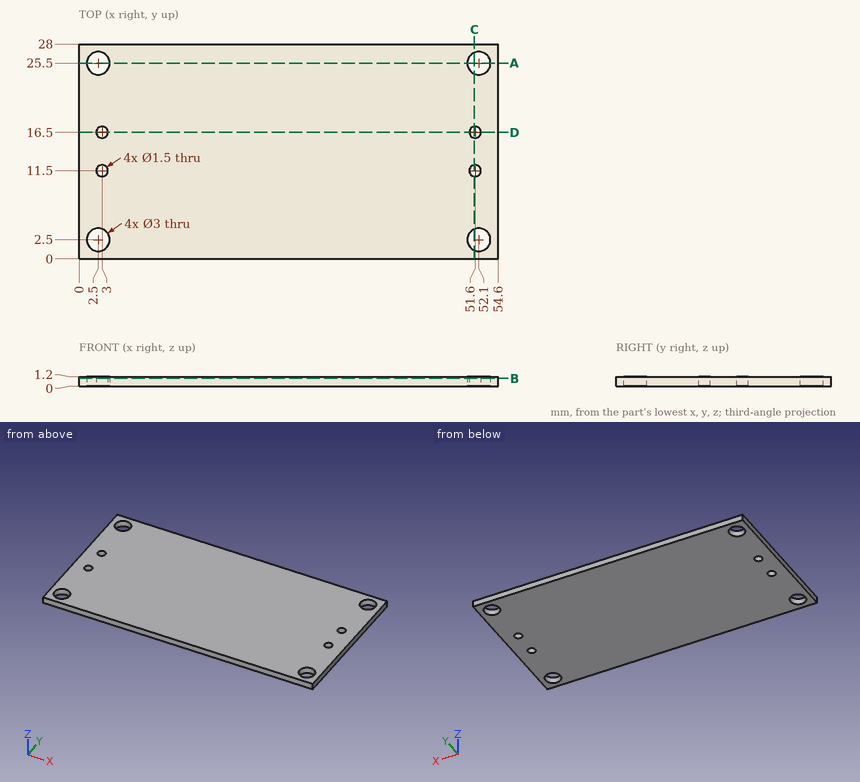
The figure shows three views and two pictorial views of one solid part (mm, origin at its lowest corner). Answer the questions. Give positions to 0.01 mm unless a question says otherwise; leave off trailing zeros. Write each loop counter-clockwise with the first axis right and the second up, starting at its lowest first coordinate (ties: lowest second). Pieces come first, ordered by that corner, then holes. Notation, with made-up numbers: (-30, 48) - (20, 48) arc R20 ccw to (20, 76) - close; hole circle Ø7 at (56.5, 14.25). An arc over 180 degrees is marked (long way). Use one line per item in the form item = value. Start each with the question number.
1) Find section A-A on y = 25.5. Determine the outline of the cut face in (x, z).
2) Find section D-D on y = 16.5. Determine the outline of the cut face in (x, z), plus the area to 3 significant figures.
3) A flat-ended cylindrical pin translates along its axis: pin 1 Ø1.8 at (x, y) = (2.5, 2.5) entering from -Z. Find the tip coordinate at first contact, or state that the pin passes through.
4) Find section C-C on x = 51.5. Determine the outline of the cut face in (y, z).
5) Consider line 1 along X through (y, z) = (16.25, 1); line 2 along X through (y, z) = (26, 0.7); line 3 along Y through (x, z) = (2.5, 0.85). Determine where each line is inside the solid, lowest interval first. Write a range as from..to.
6) Find section B-B on z = 1. Count the separate pieces of the cut face and the enclosed holes in it, plus the area to 3 significant figures.
Geometry results:
q1.outline = (0, 0) - (1, 0) - (1, 1.2) - (0, 1.2) - close; (4, 0) - (50.6, 0) - (50.6, 1.2) - (4, 1.2) - close; (53.6, 0) - (54.6, 0) - (54.6, 1.2) - (53.6, 1.2) - close
q2.outline = (0, 0) - (2.25, 0) - (2.25, 1.2) - (0, 1.2) - close; (3.75, 0) - (50.85, 0) - (50.85, 1.2) - (3.75, 1.2) - close; (52.35, 0) - (54.6, 0) - (54.6, 1.2) - (52.35, 1.2) - close
q2.area = 61.9 mm2
q3.pin_1 = through
q4.outline = (0, 0) - (1.13, 0) - (1.13, 1.2) - (0, 1.2) - close; (3.87, 0) - (10.76, 0) - (10.76, 1.2) - (3.87, 1.2) - close; (12.24, 0) - (15.76, 0) - (15.76, 1.2) - (12.24, 1.2) - close; (17.24, 0) - (24.13, 0) - (24.13, 1.2) - (17.24, 1.2) - close; (26.87, 0) - (28, 0) - (28, 1.2) - (26.87, 1.2) - close
q5.line_1 = 0..2.29, 3.71..50.89, 52.31..54.6
q5.line_2 = 0..1.09, 3.91..50.69, 53.51..54.6
q5.line_3 = 0..1, 4..10.94, 12.06..15.94, 17.06..24, 27..28
q6.separate_pieces = 1
q6.enclosed_holes = 8
q6.area = 1,490 mm2
